Autodesk Inventor part; units mm, degrees
ref_plane "YZ Plane" through (0, 0, 0) normal (1, 0, 0) x (0, 1, 0)
ref_plane "XZ Plane" through (0, 0, 0) normal (0, 1, 0) x (-1, 0, 0)
ref_plane "XY Plane" through (0, 0, 0) normal (0, 0, 1) x (1, 0, 0)
sketch "Szkic1" plane through (0, 0, 0) normal (0, 1, 0) x (-1, 0, 0)
  line L0 (0, 0) -> (-100, 0)
  line L1 (-100, 0) -> (-100, -70)
  line L2 (-100, -70) -> (0, -70)
  line L3 (0, -70) -> (0, 0)
  dimension "d0" = 100
  dimension "d1" = 70
extrude "Wyciągnięcie proste1" add sketch "Szkic1" along normal blind 0.5
sketch "Szkic2" plane through (0, 0.5, 0) normal (0, 1, 0) x (1, 0, 0)
  line L0 (84.2801, 35.4995) -> (78.4801, 35.4995)
  line L1 (84.3801, 29.5995) -> (84.3801, 35.3995)
  line L2 (78.4801, 29.4995) -> (84.2801, 29.4995)
  line L3 (78.3801, 35.3995) -> (78.3801, 29.5995)
  circle A0 centre (53.6914, 31.8917) radius 2.05
  circle A1 centre (44.8014, 31.8917) radius 2.05
  circle A2 centre (35.9114, 31.8917) radius 2.05
  line L4 (27.6783, 30.5334) -> (27.6783, 31.1734)
  line L5 (19.4183, 31.1734) -> (19.4183, 30.5334)
  line L6 (84.3801, 29.4995) -> (78.3801, 29.4995)
  line L7 (78.3801, 29.4995) -> (78.3801, 35.4995)
  line L8 (78.3801, 35.4995) -> (84.3801, 35.4995)
  line L9 (84.3801, 35.4995) -> (84.3801, 29.4995)
  line L10 (84.8801, 28.9995) -> (77.8801, 28.9995)
  line L11 (77.8801, 28.9995) -> (77.8801, 35.9995)
  line L12 (77.8801, 35.9995) -> (84.8801, 35.9995)
  line L13 (84.8801, 35.9995) -> (84.8801, 28.9995)
  circle A3 centre (53.6914, 31.8917) radius 2.55
  circle A4 centre (44.8014, 31.8917) radius 2.55
  circle A5 centre (35.9114, 31.8917) radius 2.55
  line L14 (27.6783, 30.5334) -> (19.4183, 30.5334)
  line L15 (19.4183, 30.5334) -> (19.4183, 31.1734)
  line L16 (19.4183, 31.1734) -> (27.6783, 31.1734)
  line L17 (27.6783, 31.1734) -> (27.6783, 30.5334)
  line L18 (28.9783, 32.4734) -> (18.1183, 32.4734)
  line L19 (18.1183, 32.4734) -> (18.1183, 29.2334)
  line L20 (18.1183, 29.2334) -> (28.9783, 29.2334)
  line L21 (28.9783, 29.2334) -> (28.9783, 32.4734)
  point P0 (0, 0)
  dimension "d4" = 0.5
  dimension "d5" = 0.5
  dimension "d6" = 0.5
  dimension "d7" = 0.5
  dimension "d8" = 1.3
extrude "Wyciągnięcie proste2" cut sketch "Szkic2" against normal through all contours L8 L9 L1 L6 L2 L7 L3 L0 | A0 | A1 | A2 | L14 L5 L16 L4 | L10 L11 L12 L13 | A3 | A4 | A5 | L21 L20 L19 L18
sketch "Szkic3" plane through (0, 0.5, 0) normal (0, 1, 0) x (1, 0, 0)
  circle A0 centre (3.55, 57.7319) radius 1.5
  circle A1 centre (3.55, 11.1233) radius 1.5
  circle A2 centre (96.45, 57.7319) radius 1.5
  circle A3 centre (96.45, 11.1233) radius 1.5
  circle A4 centre (25.5, 23.5) radius 1
  circle A5 centre (25.5, 14) radius 1
  circle A6 centre (50, 23.5) radius 1
  circle A7 centre (50, 14) radius 1
  circle A8 centre (74.5, 23.5) radius 1
  circle A9 centre (74.5, 14) radius 1
  point P0 (0, 0)
extrude "Wyciągnięcie proste3" cut sketch "Szkic3" against normal through all
sketch "Szkic4" plane through (0, 0.5, 0) normal (0, 1, 0) x (1, 0, 0)
  circle A0 centre (3.55, 57.7319) radius 1.5
  circle A1 centre (50, 14) radius 1
  circle A2 centre (74.5, 14) radius 1
  circle A3 centre (25.5, 23.5) radius 1
  circle A4 centre (96.45, 57.7319) radius 1.5
  circle A5 centre (3.55, 11.1233) radius 1.5
  circle A6 centre (50, 23.5) radius 1
  circle A7 centre (74.5, 23.5) radius 1
  circle A8 centre (25.5, 14) radius 1
  circle A9 centre (96.45, 11.1233) radius 1.5
  circle A10 centre (44.8014, 31.8917) radius 2.55
  circle A11 centre (35.9114, 31.8917) radius 2.55
  circle A12 centre (53.6914, 31.8917) radius 2.55
  line L0 (28.9783, 29.2334) -> (18.1183, 29.2334)
  line L1 (18.1183, 29.2334) -> (18.1183, 32.4734)
  line L2 (18.1183, 32.4734) -> (28.9783, 32.4734)
  line L3 (28.9783, 32.4734) -> (28.9783, 29.2334)
  line L4 (77.8801, 28.9995) -> (77.8801, 35.9995)
  line L5 (77.8801, 35.9995) -> (84.8801, 35.9995)
  line L6 (84.8801, 35.9995) -> (84.8801, 28.9995)
  line L7 (84.8801, 28.9995) -> (77.8801, 28.9995)
  line L8 (100, 0) -> (100, 70)
  line L9 (100, 70) -> (0, 70)
  line L10 (0, 70) -> (0, 0)
  line L11 (0, 0) -> (100, 0)
extrude "Wyciągnięcie proste4" add sketch "Szkic4" along normal blind 1.2
sketch "Szkic5" plane through (0, 1.7, 0) normal (0, 1, 0) x (1, 0, 0)
  circle A0 centre (25.5, 14) radius 1
  line L0 (100, 70) -> (0, 70)
  line L1 (0, 70) -> (0, 0)
  line L2 (0, 0) -> (100, 0)
  line L3 (100, 0) -> (100, 70)
  circle A1 centre (53.6914, 31.8917) radius 2.55
  circle A2 centre (44.8014, 31.8917) radius 2.55
  circle A3 centre (25.5, 14) radius 1
  circle A4 centre (3.55, 57.7319) radius 1.5
  circle A5 centre (50, 14) radius 1
  circle A6 centre (74.5, 14) radius 1
  circle A7 centre (25.5, 23.5) radius 1
  circle A8 centre (96.45, 57.7319) radius 1.5
  circle A9 centre (3.55, 11.1233) radius 1.5
  circle A10 centre (50, 23.5) radius 1
  circle A11 centre (74.5, 23.5) radius 1
  circle A12 centre (96.45, 11.1233) radius 1.5
  circle A13 centre (35.9114, 31.8917) radius 2.55
  line L4 (77.8801, 28.9995) -> (77.8801, 35.9995)
  line L5 (77.8801, 35.9995) -> (84.8801, 35.9995)
  line L6 (84.8801, 35.9995) -> (84.8801, 28.9995)
  line L7 (84.8801, 28.9995) -> (77.8801, 28.9995)
  line L8 (28.9783, 29.2334) -> (18.1183, 29.2334)
  line L9 (18.1183, 29.2334) -> (18.1183, 32.4734)
  line L10 (18.1183, 32.4734) -> (28.9783, 32.4734)
  line L11 (28.9783, 32.4734) -> (28.9783, 29.2334)
  circle A14 centre (3.55, 11.1233) radius 1.5
  circle A15 centre (3.55, 11.1233) radius 1.75
  circle A16 centre (3.55, 57.7319) radius 1.5
  circle A17 centre (3.55, 57.7319) radius 1.75
  circle A18 centre (96.45, 11.1233) radius 1.75
  circle A19 centre (96.45, 57.7319) radius 1.5
  circle A20 centre (96.45, 57.7319) radius 1.75
  circle A21 centre (25.5, 14) radius 1
  circle A22 centre (25.5, 14) radius 1.25
  circle A23 centre (25.5, 23.5) radius 1
  circle A24 centre (25.5, 23.5) radius 1.25
  circle A25 centre (50, 23.5) radius 1
  circle A26 centre (50, 23.5) radius 1.25
  circle A27 centre (50, 14) radius 1
  circle A28 centre (50, 14) radius 1.25
  circle A29 centre (74.5, 23.5) radius 1
  circle A30 centre (74.5, 23.5) radius 1.25
  circle A31 centre (74.5, 14) radius 1
  circle A32 centre (74.5, 14) radius 1.25
  dimension "d15" = 3.5
  dimension "d16" = 3.5
  dimension "d17" = 3.5
  dimension "d18" = 3.5
  dimension "d19" = 2.5
  dimension "d20" = 2.5
  dimension "d21" = 2.5
  dimension "d22" = 2.5
  dimension "d23" = 2.5
  dimension "d24" = 2.5
extrude "Wyciągnięcie proste5" cut sketch "Szkic5" against normal through all contours A0 | A4 | A5 | A6 | A7 | A8 | A9 | A10 | A11 | A12 | A15 | A17 | A18 | A20 | A22 | A24 | A26 | A28 | A30 | A32
sketch "Szkic6" plane through (0, 1.7, 0) normal (0, 1, 0) x (1, 0, 0)
  circle A0 centre (50, 23.5) radius 1.25
  circle A1 centre (50, 14) radius 1.25
  circle A2 centre (50, 14) radius 1.25
  line L0 (50, 23.5) -> (50, 14) construction
  line L1 (52, 23.5) -> (52, 14)
  line L2 (48, 14) -> (48, 23.5)
  arc A3 (52, 23.5) -> (48, 23.5) centre (50, 23.5) ccw
  arc A4 (48, 14) -> (52, 14) centre (50, 14) ccw
  point P0 (0, 0)
  point P1 (50, 18.75)
extrude "Wyciągnięcie proste6" cut sketch "Szkic6" against normal through all contours A0 | A1 | L1 A4 L2 A3
sketch "Szkic7" plane through (0, 1.7, 0) normal (0, 1, 0) x (1, 0, 0)
  arc A0 (52, 23.5) -> (48, 23.5) centre (50, 23.5) ccw
  line L0 (52, 23.5) -> (52, 14)
  arc A1 (48, 14) -> (52, 14) centre (50, 14) ccw
  line L1 (48, 14) -> (48, 23.5)
  circle A2 centre (25.5, 23.5) radius 1.25
  circle A3 centre (74.5, 23.5) radius 1.25
  circle A4 centre (96.45, 57.7319) radius 1.75
  circle A5 centre (3.55, 11.1233) radius 1.75
  circle A6 centre (25.5, 14) radius 1.25
  circle A7 centre (74.5, 14) radius 1.25
  circle A8 centre (96.45, 11.1233) radius 1.75
  circle A9 centre (3.55, 57.7319) radius 1.75
  line L2 (100, 70) -> (0, 70)
  line L3 (0, 70) -> (0, 0)
  line L4 (0, 0) -> (100, 0)
  line L5 (100, 0) -> (100, 70)
  circle A10 centre (53.6914, 31.8917) radius 2.55
  circle A11 centre (44.8014, 31.8917) radius 2.55
  circle A12 centre (35.9114, 31.8917) radius 2.55
  line L6 (77.8801, 28.9995) -> (77.8801, 35.9995)
  line L7 (77.8801, 35.9995) -> (84.8801, 35.9995)
  line L8 (84.8801, 35.9995) -> (84.8801, 28.9995)
  line L9 (84.8801, 28.9995) -> (77.8801, 28.9995)
  line L10 (28.9783, 29.2334) -> (18.1183, 29.2334)
  line L11 (18.1183, 29.2334) -> (18.1183, 32.4734)
  line L12 (18.1183, 32.4734) -> (28.9783, 32.4734)
  line L13 (28.9783, 32.4734) -> (28.9783, 29.2334)
extrude "Wyciągnięcie proste7" add sketch "Szkic7" along normal blind 0.3
sketch "Szkic8" plane through (0, 2, 0) normal (0, 1, 0) x (1, 0, 0)
  line L0 (0, 0) -> (100, 0)
  line L1 (100, 0) -> (0, 0)
  line L2 (0, 0) -> (0, -2)
  line L3 (0, -2) -> (100, -2)
  line L4 (100, -2) -> (100, 0)
  dimension "d31" = 2
extrude "Wyciągnięcie proste8" add sketch "Szkic8" against normal blind 2
sketch "Szkic9" plane through (0, 2, 0) normal (0, 1, 0) x (1, 0, 0)
  line L0 (28.9783, 32.4734) -> (28.9783, 29.2334)
  line L1 (18.1183, 29.2334) -> (18.1183, 32.4734)
  line L2 (18.1183, 32.4734) -> (28.9783, 32.4734)
  line L3 (28.9783, 29.2334) -> (18.1183, 29.2334)
  line L4 (18.1183, 30.8534) -> (28.9783, 30.8534) construction
  line L5 (19.7383, 32.4734) -> (27.3583, 32.4734)
  line L6 (27.3583, 29.2334) -> (19.7383, 29.2334)
  arc A0 (19.7383, 32.4734) -> (19.7383, 29.2334) centre (19.7383, 30.8534) ccw
  arc A1 (27.3583, 29.2334) -> (27.3583, 32.4734) centre (27.3583, 30.8534) ccw
  point P0 (0, 0)
  point P1 (23.5483, 30.8534)
extrude "Wyciągnięcie proste9" add sketch "Szkic9" against normal up to surface (2 mm away) contours L0 A1 L2 | L0 L3 A1 | A0 L1 L2 | L3 L1 A0
sketch "Szkic10" plane through (0, 2, 0) normal (0, 1, 0) x (1, 0, 0)
  line L0 (77.8801, 35.9995) -> (84.8801, 35.9995)
  line L1 (84.8801, 35.9995) -> (84.8801, 28.9995)
  line L2 (84.8801, 28.9995) -> (77.8801, 28.9995)
  line L3 (77.8801, 28.9995) -> (77.8801, 35.9995)
  circle A0 centre (81.3801, 32.4995) radius 2.5
  point P0 (0, 0)
  dimension "d36" = 5
extrude "Wyciągnięcie proste10" add sketch "Szkic10" against normal up to surface (2 mm away)
sketch "Szkic11" plane through (0, 2, 0) normal (0, 1, 0) x (1, 0, 0)
  line L0 (19.7383, 32.4734) -> (27.3583, 32.4734)
  arc A0 (27.3583, 29.2334) -> (27.3583, 32.4734) centre (27.3583, 30.8534) ccw
  line L1 (27.3583, 29.2334) -> (19.7383, 29.2334)
  arc A1 (19.7383, 32.4734) -> (19.7383, 29.2334) centre (19.7383, 30.8534) ccw
  circle A2 centre (19.7383, 30.8534) radius 1.62
  circle A3 centre (27.3583, 30.8534) radius 1.62
  circle A4 centre (23.5483, 30.8534) radius 1.62
  point P0 (0, 0)
  point P1 (23.5483, 29.2334)
  point P2 (23.5483, 32.4734)
extrude "Wyciągnięcie proste11" add sketch "Szkic11" against normal up to surface (2 mm away) contours L0 A4 L1 A2 | L0 A3 L1 A4
sketch "Szkic12" plane through (0, 2, 0) normal (0, 1, 0) x (1, 0, 0)
  arc A0 (52, 23.5) -> (48, 23.5) centre (50, 23.5) ccw
  line L0 (52, 23.5) -> (52, 14)
  line L1 (48, 14) -> (48, 23.5)
  arc A1 (48, 14) -> (52, 14) centre (50, 14) ccw
  arc A2 (53, 23.5) -> (47, 23.5) centre (50, 23.5) ccw
  line L2 (53, 23.5) -> (53, 14)
  arc A3 (47, 14) -> (53, 14) centre (50, 14) ccw
  line L3 (47, 14) -> (47, 23.5)
  point P0 (0, 0)
extrude "Wyciągnięcie proste12" cut sketch "Szkic12" against normal through all contours L0 A1 L1 A0 | L2 A3 L3 A2
properties part number "dach" material "Stal miękka, spawana"
The model under review builds one solid part; all positions refer to its coordinate system, in mm. A direction names the side the tool comes from. Round coordinates to 2 decimals unless told otherwise and drop trailing zeros. Loops run counter-clockwise (first coordinate to the right, second up) from the corner with the lowest first, then second, coordinate; pieces in that order, holes last. Notation, with made-up numbers: (-21.75, 29) -> (26.25, 29) arc R3 cw to (26.25, 34) -> close; hole circle Ø11 at (56.5, -32). An arc over 180 degrees is marked (long way). Answer as a JSON object with one key per item and string values. Group by question number.
1) For pin 1 Ø4.5 at (x, z) = (35.91, -31.89) entering from +Y, flat-tipped, find the tip position at first contact; note if it passes through.
2) Mouldability with a two-part tool opening along X and no side actions: class faces 3 (the face through (100, 1, -33)), 4 (the face through (49, 0, -35)), 5 (the face through (50, 1, -11)) as released by +X, released by -X, zero draft, split by the parting line, or undercut.
3) We need section D-D on x = 3.55. Write out the cut boundary in (y, z), then the cut area to 3 significant figures.
4) For faces 1 (the face through (0, 1, -35)), 2 (the face through (53, 1, -19)), list the 3-axis set-ups (+Z, -Z, +X, -X, +Y, -Y) from which the entire face can be reached by the end or side of a thin tool; tool diameter is ignored.
5) We need section B-B on x = 34.5. Write out the cut boundary in (y, z).
6) For line 1 (Z direction, x = 74.5, y = 1.5); line 2 (Z direction, x = 3.55, y = 0.5); line 3 (X direction, y = 1.2, z = -59), list the stretches that pass through material, from the lowest coordinate up. Write a range as [from, to].
7) We need section C-C on y = 1.1. Give the number of separate pieces and of enclosed holes in the cut face, then the cut area to 3 significant figures.
8) We need section A-A on x = 74.5. Write out the cut boundary in (y, z).
Result set:
{
 "1": {"pin 1": "through"},
 "2": {"face 3": "released by +X", "face 4": "zero draft", "face 5": "undercut"},
 "3": {"outline": "(0, -70) -> (2, -70) -> (2, -59.48) -> (0, -59.48) -> close; (0, -55.98) -> (2, -55.98) -> (2, -12.87) -> (0, -12.87) -> close; (0, -9.37) -> (2, -9.37) -> (2, 2) -> (0, 2) -> close", "area": "130 mm²"},
 "4": {"face 1": "+Z, -Z, -X, +Y, -Y", "face 2": "+Y, -Y"},
 "5": {"outline": "(0, -70) -> (2, -70) -> (2, -34.02) -> (0, -34.02) -> close; (0, -29.77) -> (2, -29.77) -> (2, 2) -> (0, 2) -> close"},
 "6": {"line 1": "[-70, -24.75], [-22.25, -15.25], [-12.75, 2]", "line 2": "[-70, -59.48], [-55.98, -12.87], [-9.37, 2]", "line 3": "[0, 2.34], [4.76, 95.24], [97.66, 100]"},
 "7": {"separate pieces": "1", "enclosed holes": "16", "area": "6,950 mm²"},
 "8": {"outline": "(0, -70) -> (2, -70) -> (2, -24.75) -> (0, -24.75) -> close; (0, -22.25) -> (2, -22.25) -> (2, -15.25) -> (0, -15.25) -> close; (0, -12.75) -> (2, -12.75) -> (2, 2) -> (0, 2) -> close"}
}
